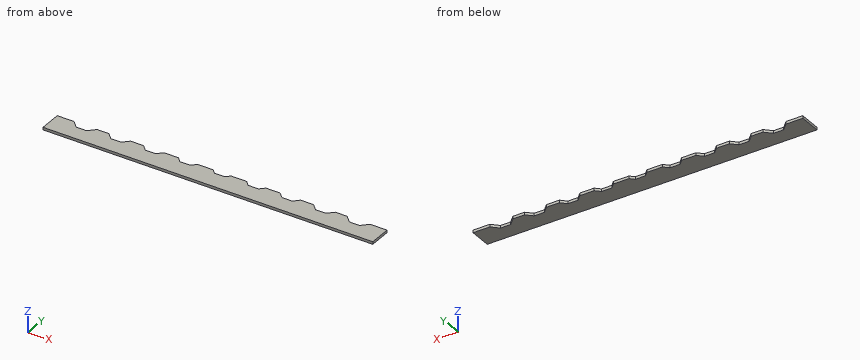
```python
from build123d import *

# Parameters (mm, degrees)
SKETCH1_W             = 1285
SKETCH1_H             = 85
BOSS_EXTRUDE1_DEPTH   = 10
CUT_EXTRUDE1_REACH    = 650.175
SKETCH_PATTERN1_DEPTH = 10


# Read off the part's stored shape, not the designer's step: Sketch-Pattern1
with BuildPart() as part:
    # Sketch1 → Boss-Extrude1 (new body)
    with BuildSketch(Plane.XY):
        with Locations((0, 42.5)):
            Rectangle(SKETCH1_W, SKETCH1_H)
    extrude(amount=BOSS_EXTRUDE1_DEPTH)

    # Sketch2 → Cut-Extrude1 (cut, up to next)
    with BuildSketch(Plane.XY.offset(10), mode=Mode.PRIVATE) as cut_extrude1_sk1:
        Polygon((-50, 100), (-20, 70), (20, 70), (50, 100), align=None)
    cut_extrude1_tool1 = extrude(cut_extrude1_sk1.sketch, amount=-CUT_EXTRUDE1_REACH, mode=Mode.PRIVATE) & part.part
    add(cut_extrude1_tool1.solids().sort_by_distance((0, 87.142857, 10))[0], mode=Mode.SUBTRACT)

    # Sketch-Pattern1 outline → Sketch-Pattern1 (cut)
    with BuildSketch(Plane.XY):
        Polygon((-286, 65), (-246, 65), (-226, 85), (-306, 85), align=None)
        Polygon((-512, 60), (-487, 85), (-577, 85), (-552, 60), align=None)
        Polygon((-379, 62.5), (-356.5, 85), (-441.5, 85), (-419, 62.5), align=None)
        Polygon((-95.5, 85), (-170.5, 85), (-153, 67.5), (-113, 67.5), align=None)
    sketch_pattern1 = extrude(amount=SKETCH_PATTERN1_DEPTH, mode=Mode.SUBTRACT)

    # Mirror1: Sketch-Pattern1 across plane
    add(sketch_pattern1.mirror(Plane(origin=(0, 0, 0), x_dir=(0, 0, 1), z_dir=(1, 0, 0))), mode=Mode.SUBTRACT)


solid = part.part
```
The model under review builds one solid part; all positions refer to its coordinate system, in mm. Round coordinates to 2 decimals unless told otherwise and drop trailing zeros. Write each loop counter-clockwise with the first axis right and the second up, starting at its lowest first coordinate (ties: lowest second). Pieces come first, ordered by that corner, then holes. Notation, with made-up numbers: (33, 75) -> (81, 75) arc R30 ccw to (81, 101) -> close; hole circle Ø11 at (61.25, -30.5). An arc over 180 degrees is marked (long way). Use CSV: the item, a comma, the result in double quotes.
Q1. Consider section A-A (x = -5.5). Give the boundary of the cut face in (y, z), then the cut area to 3 significant figures.
Checks:
outline,"(0, 0) -> (70, 0) -> (70, 10) -> (0, 10) -> close"
area,"700 mm²"
Q2. To check wall thickness, follow probe 1 along X at (y, z) = (61.5, 6.75); probe 2 along Y at (x, z) = (538, 1); probe 3 along Y at (x, z) = (-505.5, 6). State the ranges of each line that lie inside material, in increasing order. Write a range as [from, to].
Checks:
probe 1,"[-642.5, -553.5], [-510.5, 510.5], [553.5, 642.5]"
probe 2,"[0, 60]"
probe 3,"[0, 66.5]"
Q3. Consider section B-B (x = 538). Give the boundary of the cut face in (y, z).
Checks:
outline,"(0, 0) -> (60, 0) -> (60, 10) -> (0, 10) -> close"
Q4. For pin 1 Ø5 at (x, z) = (-407.5, 6) entering from +Y; pin 2 Ø5 at (x, z) = (-531.5, 2.5) entering from +Y; pin 3 Ø3 at (x, z) = (138.5, 3.5) entering from +Y, all flat-tipped, find the tip position at first contact; note any pin that passes through.
Checks:
pin 1,"y = 62.5"
pin 2,"y = 60"
pin 3,"y = 67.5"
